Can you work these out from the model? Positions are in its coordinate system, mm. Coordinates: 2 decimals unless noted, no trailing zeros. Use one line per item in the form item = value. Start each with the question number.
(1) Imagine slicing it at A-A (y = 4.5). State how many separate pieces and enclosed holes the cut face has, plus the area to 3 significant figures.
(2) I need wall thicknesses on line 1 (X direction, y = 4.25, z = 609.6); line 2 (Z direction, x = 508, y = 2.5); line 3 (X direction, y = 2.5, z = -685.8). Which ranges of each line are inside material? Lowest first, please. Write a range as [from, to].
(3) I'm going to push a flat-ended pin straight in: pin 1 (15 mm diameter, centred on x = 233.49, z = 685.8, fed in from +Y). Where does the tip first touch, or does it pass through?
```python
from build123d import *

# Parameters (mm, degrees)
SKETCH1_W               = 1219.2
SKETCH1_H               = 1524
BOSS_EXTRUDE1_DEPTH     = 6.35
SKETCH20_R              = 1360.3436129
SKETCH20_R_2            = 1357.8036129
CUT_EXTRUDE_THIN2_DEPTH = 6.35
SKETCH24_R              = 4.7625
CUT_EXTRUDE13_DEPTH     = 976.856794053


with BuildPart() as part:
    # Sketch1 → Boss-Extrude1 (new body)
    with BuildSketch(Plane(origin=(0, 0, 0), x_dir=(1, 0, 0), z_dir=(0, 1, 0))):
        Rectangle(SKETCH1_W, SKETCH1_H)
    extrude(amount=BOSS_EXTRUDE1_DEPTH)

    # Sketch20 → Cut-Extrude-Thin2 (cut)
    with BuildSketch(Plane(origin=(0, 6.35, 0), x_dir=(1, 0, 0), z_dir=(0, 1, 0))):
        Circle(SKETCH20_R)
        Circle(SKETCH20_R_2, mode=Mode.SUBTRACT)
        Polygon((612.14, -610.652102448), (458.252102448, -764.54), (0, -764.54), (-458.252102448, -764.54), (-612.14, -610.652102448), (-612.14, 610.652102448), (-458.252102448, 764.54), (0, 764.54), (458.252102448, 764.54), (612.14, 610.652102448), align=None)
        Polygon((609.6, -609.6), (457.2, -762), (0, -762), (-457.2, -762), (-609.6, -609.6), (-609.6, 609.6), (-457.2, 762), (0, 762), (457.2, 762), (609.6, 609.6), align=None, mode=Mode.SUBTRACT)
    extrude(amount=-CUT_EXTRUDE_THIN2_DEPTH, mode=Mode.SUBTRACT)


with BuildPart() as cut_extrude_thin2_kept_piece:
    # of the separate pieces the step leaves, the one the design keeps (cut_extrude_thin2_pieces_kept)
    add(part.part.solids().sort_by_distance((457.2, 6.35, -762))[0])

    # Sketch24 → Cut-Extrude13 (cut, through all)
    with BuildSketch(Plane.XZ):
        with Locations(Location((-279.400040578, -0.001758284, 0), (0, 0, 270))):
            Circle(SKETCH24_R)
        with Locations(Location((-279.400040578, 165.098241716, 0), (0, 0, 270))):
            Circle(SKETCH24_R)
        with Locations(Location((-279.400040578, 330.198241716, 0), (0, 0, 270))):
            Circle(SKETCH24_R)
        with Locations(Location((-279.400040578, 495.298241716, 0), (0, 0, 270))):
            Circle(SKETCH24_R)
        with Locations(Location((87.436757408, 685.8, 0), (0, 0, 270))):
            Circle(SKETCH24_R)
        with Locations(Location((233.486757408, 685.8, 0), (0, 0, 270))):
            Circle(SKETCH24_R)
        with Locations(Location((284.709719006, 495.298241716, 0), (0, 0, 270))):
            Circle(SKETCH24_R)
        with Locations(Location((284.709719006, 330.198241716, 0), (0, 0, 270))):
            Circle(SKETCH24_R)
        with Locations(Location((284.709719006, 165.098241716, 0), (0, 0, 270))):
            Circle(SKETCH24_R)
        with Locations(Location((284.709719006, -0.001758284, 0), (0, 0, 270))):
            Circle(SKETCH24_R)
        with Locations(Location((284.709719006, -165.101758284, 0), (0, 0, 270))):
            Circle(SKETCH24_R)
        with Locations(Location((284.709719006, -330.201758284, 0), (0, 0, 270))):
            Circle(SKETCH24_R)
        with Locations(Location((284.709719006, -495.301758284, 0), (0, 0, 270))):
            Circle(SKETCH24_R)
        with Locations(Location((233.486757408, -685.8, 0), (0, 0, 270))):
            Circle(SKETCH24_R)
        with Locations(Location((87.436757408, -685.8, 0), (0, 0, 270))):
            Circle(SKETCH24_R)
        with Locations(Location((-58.613242592, -685.8, 0), (0, 0, 270))):
            Circle(SKETCH24_R)
        with Locations(Location((-204.663242592, -685.8, 0), (0, 0, 270))):
            Circle(SKETCH24_R)
        with Locations(Location((-279.400040578, -495.301758284, 0), (0, 0, 270))):
            Circle(SKETCH24_R)
        with Locations(Location((-279.400040578, -330.201758284, 0), (0, 0, 270))):
            Circle(SKETCH24_R)
        with Locations(Location((-279.400040578, -165.101758284, 0), (0, 0, 270))):
            Circle(SKETCH24_R)
        with Locations(Location((508, -609.6, 0), (0, 0, 270))):
            Circle(SKETCH24_R)
        with Locations(Location((508, 609.6, 0), (0, 0, 270))):
            Circle(SKETCH24_R)
        with Locations(Location((-508, -609.6, 0), (0, 0, 270))):
            Circle(SKETCH24_R)
        with Locations(Location((-508, 609.6, 0), (0, 0, 270))):
            Circle(SKETCH24_R)
        with Locations(Location((-204.663242592, 685.8, 0), (0, 0, 270))):
            Circle(SKETCH24_R)
        with Locations(Location((-58.613242592, 685.8, 0), (0, 0, 270))):
            Circle(SKETCH24_R)
        with Locations(Location((-508, 0, 0), (0, 0, 270))):
            Circle(SKETCH24_R)
        with Locations(Location((508, 0, 0), (0, 0, 270))):
            Circle(SKETCH24_R)
    extrude(amount=-CUT_EXTRUDE13_DEPTH, mode=Mode.SUBTRACT)


solid = cut_extrude_thin2_kept_piece.part
```
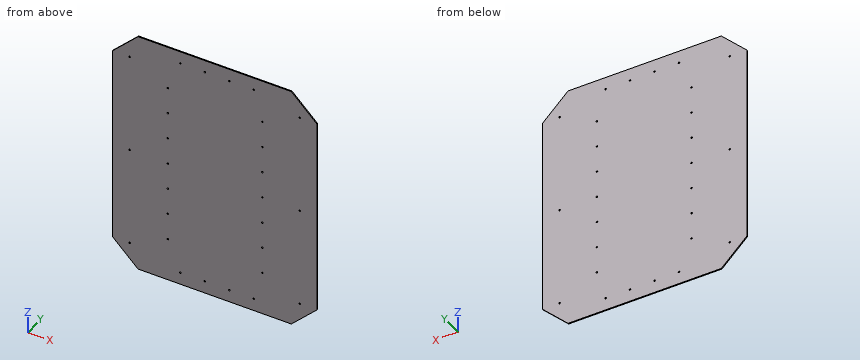
Worked out:
q1.separate_pieces = 1
q1.enclosed_holes = 28
q1.area = 1,810,000 mm2
q2.line_1 = [-609.6, -512.76], [-503.24, 503.24], [512.76, 609.6]
q2.line_2 = [-711.2, -614.36], [-604.84, -4.76], [4.76, 604.84], [614.36, 711.2]
q2.line_3 = [-533.4, -209.43], [-199.9, -63.38], [-53.85, 82.67], [92.2, 228.72], [238.25, 533.4]
q3.pin_1 = 6.35
